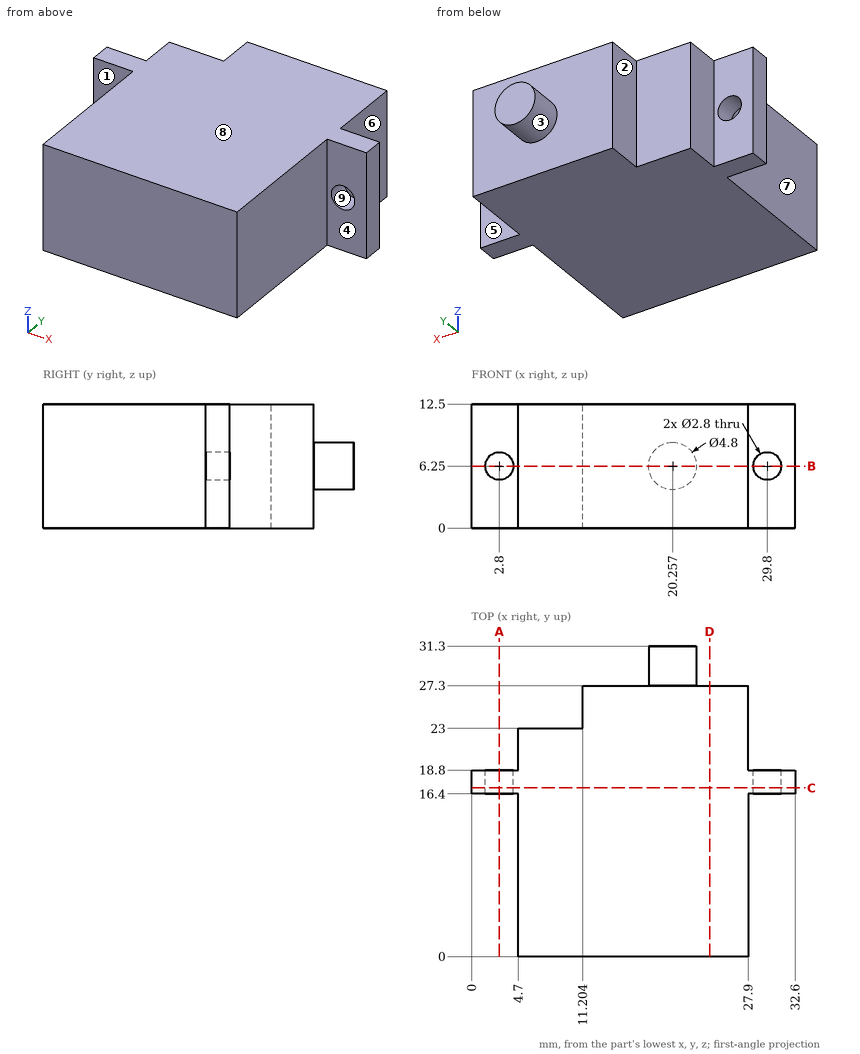
Source: three-view drawing plus pictorial views. Frame: mm from the lowest corner of the part. A direction names the side the tool comes from. Give positions to 0.01 mm unless a question says otherwise; leave off trailing zeros. Loops run counter-clockwise (first coordinate to the right, second up) from the corner with the lowest first, then second, coordinate; pieces in that order, holes last. Notation, with made-up numbers: (-23.75, 37) -> (-8.75, 37) arc R25 ccw to (-8.75, 52) -> close; hole circle Ø3 at (-40, 16.25). An arc over 180 degrees is marked (long way). Use a Markdown table: item, result. Add a question column.
(1) Ray query, line 1 (X direction, y = 17, z = 6.25); line 2 (Y direction, x = 15, z = 5.5); line 3 (Z direction, x = 2, y = 17). Return the intervals inside material, ascending.
(2) Access query for the marked faces 1, 2, 3, 4 and 5. Directions: +Z, -Z, +X, -X, +Y, -Y. A direction counts if a zero-diameter tool reaches every point of the face in a straight line with its end or side. Return the directions, or none.
(3) Section query B-B (z = 6.25). Output: boundary loops of the cut face in (x, y), then the cut area to 3 significant figures.
(4) Section query A-A (x = 2.8). Output: boundary loops of the cut face in (y, z).
(5) Section query D-D (x = 24). Output: boundary loops of the cut face in (y, z), then the cut area to 3 significant figures.
(6) First-contact query: pin 1 Ø7 at (x, z) = (9.5, 9) entering from +Y; pin 2 Ø1.4 at (x, z) = (3, 7.5) entering from +Y; pin 3 Ø2.5 at (y, z) = (23, 5.5) entering from +X. Flat tips, straight axial feed; report the tip coordinate or a pass-through.
(7) Section query C-C (y = 17). Output: boundary loops of the cut face in (x, z).
(8) Pull-direction query (X, two-part tool) for the marked faces 6, 7, 8 and 9; classes: +X half, -X half, draft (parallel to the pull), parting line (faces both ways), or undercut.
Checked values:
| question | item | result |
|---|---|---|
| 1 | line 1 | 0 to 1.4, 4.2 to 28.4, 31.2 to 32.6 |
| 1 | line 2 | 0 to 27.3 |
| 1 | line 3 | 0 to 5.1, 7.4 to 12.5 |
| 2 | face 1 | +Z, -Z, -X, -Y |
| 2 | face 2 | +Z, -Z, -X, +Y |
| 2 | face 3 | +Y |
| 2 | face 4 | +Z, -Z, +X, -Y |
| 2 | face 5 | +Z, -Z, +X, +Y |
| 3 | outline | (0, 16.4) -> (1.4, 16.4) -> (1.4, 18.8) -> (0, 18.8) -> close; (4.2, 16.4) -> (4.7, 16.4) -> (4.7, 0) -> (27.9, 0) -> (27.9, 16.4) -> (28.4, 16.4) -> (28.4, 18.8) -> (27.9, 18.8) -> (27.9, 27.3) -> (22.66, 27.3) -> (22.66, 31.3) -> (17.86, 31.3) -> (17.86, 27.3) -> (11.2, 27.3) -> (11.2, 23) -> (4.7, 23) -> (4.7, 18.8) -> (4.2, 18.8) -> close; (31.2, 16.4) -> (32.6, 16.4) -> (32.6, 18.8) -> (31.2, 18.8) -> close |
| 3 | area | 634 mm^2 |
| 4 | outline | (16.4, 0) -> (18.8, 0) -> (18.8, 4.85) -> (16.4, 4.85) -> close; (16.4, 7.65) -> (18.8, 7.65) -> (18.8, 12.5) -> (16.4, 12.5) -> close |
| 5 | outline | (0, 0) -> (27.3, 0) -> (27.3, 12.5) -> (0, 12.5) -> close |
| 5 | area | 341 mm^2 |
| 6 | pin 1 | y = 27.3 |
| 6 | pin 2 | y = 18.8 |
| 6 | pin 3 | x = 27.9 |
| 7 | outline | (0, 0) -> (32.6, 0) -> (32.6, 12.5) -> (0, 12.5) -> close; hole circle Ø2.8 at (2.8, 6.25); hole circle Ø2.8 at (29.8, 6.25) |
| 8 | face 6 | +X half |
| 8 | face 7 | -X half |
| 8 | face 8 | draft |
| 8 | face 9 | undercut |
